Answer from the drawing. Dimensions are ordinates in mm from the lowest x, y and z of the part. A direction names the side the tool comes from. Coordinates: 2 decimals unless noted, no trailing zeros. Order: outer loops, then holes, each group sorted by start corner. A loop starts at its lowest first (then second) coordinate and runs counter-clockwise, first axis right, second up. Notation, with made-up numbers: (-2.75, -34) - (17.25, -34) arc R32 cw to (17.25, 5) - close; hole circle Ø10 at (-9.5, 1). An arc over 180 degrees is marked (long way). One line per item, written item: value. Start each with the question number.
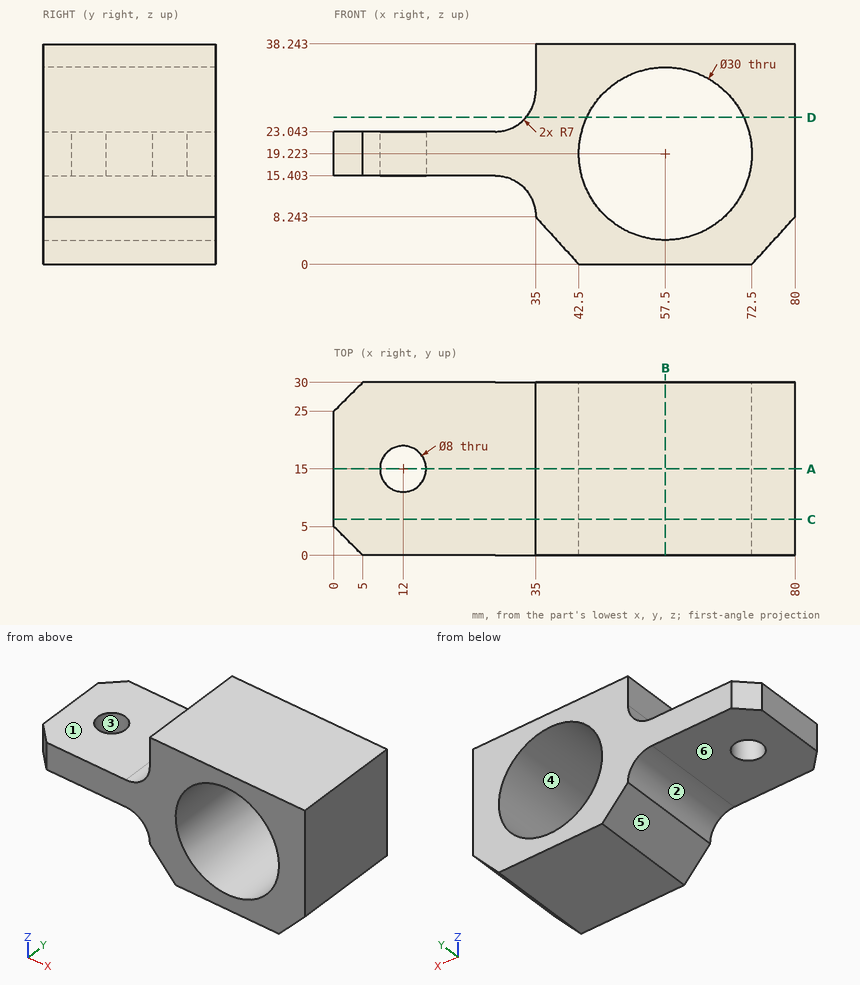
(1) The part is cut by section C-C on y = 6.25. Determine the outline of the cut face in (x, z).
(2) For the marked faces 1 and 2, determine the directions among +Z, -Z, +X, -X, +Y, -Y from which every point of the face is accessible in a straight line to the end or side of a thin tool.
(3) Flat-ended cylindrical pins translate along their axes: pin 1 Ø2.5 at (y, z) = (19.5, 32.5) entering from -X; pin 2 Ø1 at (x, y) = (64, 18.5) entering from -Z; pin 3 Ø9 at (x, y) = (12, 15) entering from -Z. Find the tip coordinate at first contact, or state that the pin passes through.
(4) The part is cut by section D-D on z = 25.5. Determine the outline of the cut face in (x, y) (1 decimal), plus the area to 3 significant figures.
(5) Consider probe 1 along X at (y, z) = (12.5, 6.5) (1 decimal); probe 2 along X at (y, z) = (1.5, 27) (1 decimal); probe 3 along Z at (x, y) = (26, 8.5). Determine where each line is inside the solid, lowest interval first.
(6) For a pull along X with two mould halves and no side action, classify the marked faces 3, 4, 5 and 6 as pulls with the +X half, pulls with the -X half, needs draft (parallel to the pull), parting line crosses it, or undercut.
(7) The part is cut by section B-B on x = 57.5. Determine the outline of the cut face in (y, z).
(8) The part is cut by section A-A on y = 15. Determine the outline of the cut face in (x, z).
Completed:
1. outline: (0, 15.4) - (28, 15.4) arc R7 cw to (35, 8.4) - (35, 8.24) - (42.5, 0) - (72.5, 0) - (80, 8.24) - (80, 38.24) - (35, 38.24) - (35, 30.04) arc R7 cw to (28, 23.04) - (0, 23.04) - close; hole circle Ø30 at (57.5, 19.22)
2. face 1: +Z, -X, +Y, -Y
2. face 2: -Z, -X, +Y, -Y
3. pin 1: stops at x = 35
3. pin 2: stops at z = 0
3. pin 3: stops at z = 15.4
4. outline: (33.3, 0) - (43.9, 0) - (43.9, 30) - (33.3, 30) - close; (71.1, 0) - (80, 0) - (80, 30) - (71.1, 30) - close
4. area: 583 mm2
5. probe 1: x = 36.6 to 49.6, 65.4 to 78.4
5. probe 2: x = 34.3 to 44.7, 70.3 to 80
5. probe 3: z = 15.4 to 23.04
6. face 3: undercut
6. face 4: undercut
6. face 5: pulls with the -X half
6. face 6: needs draft
7. outline: (0, 0) - (30, 0) - (30, 4.22) - (0, 4.22) - close; (0, 34.22) - (30, 34.22) - (30, 38.24) - (0, 38.24) - close
8. outline: (0, 15.4) - (8, 15.4) - (8, 23.04) - (0, 23.04) - close; (16, 15.4) - (28, 15.4) arc R7 cw to (35, 8.4) - (35, 8.24) - (42.5, 0) - (72.5, 0) - (80, 8.24) - (80, 38.24) - (35, 38.24) - (35, 30.04) arc R7 cw to (28, 23.04) - (16, 23.04) - close; hole circle Ø30 at (57.5, 19.22)
